Could you check a few things on this model? Use its own coordinates, in mm. Face numbers are marked on the shaded views. A direction names the side the tool comes from. Coordinates: 2 decimals unless noted, no trailing zeros. Order: outer loops, then holes, each group sorted by start corner. A loop starts at its lowest first (then second) coordinate and runs counter-clockwise, first axis right, second up. Notation, with made-up numbers: (42, 70.25) -> (70, 70.25) arc R17 ccw to (70, 98.25) -> close; hole circle Ø10 at (52.5, -36.5). An arc over 180 degrees is marked (long way). Put each result on its own line as item: value. Start each with the question number.
Q1. For the marked faces 1 and 2, which set-ups out of +Z, -Z, +X, -X, +Y, -Y let a thin tool reach every point of the face, with its end or its side?
Q2. We'd pull the mould along Y, two halves only. Please class the marked faces 3, 4 and 5: +Y half, -Y half, draft (parallel to the pull), parting line (faces both ways), or undercut.
Q3. If we section it at C-C (y = 27): Please give me the cut outline in (x, z) (3 decimals).
Q4. If we section it at B-B (x = 0): Please give me the cut outline in (y, z) (3 decimals), and give its area (3 significant figures).
Q5. Will these pins go through, and if not, where does the flat tip stop? pin 1 (1 mm diameter, centred on y = 61.5, z = 20, fed in from +X); pin 2 (4 mm diameter, centred on y = 29, z = 8, fed in from +X); pin 3 (7.5 mm diameter, centred on x = 0, y = 90.49, fed in from +Z); pin 4 (9 mm diameter, centred on x = 0, z = 0, fed in from -Y).
Q6. If we section it at A-A (z = 0): Please give me the cut outline in (x, y) (3 decimals), and give its area (3 significant figures).
Q7. Please list where these lines run through material, in increasing order: line 1 along Y through (x, z) = (0, -9) (3 decimals); line 2 along Z through (x, y) = (0, 77); line 3 along Z through (x, y) = (-6, 31).
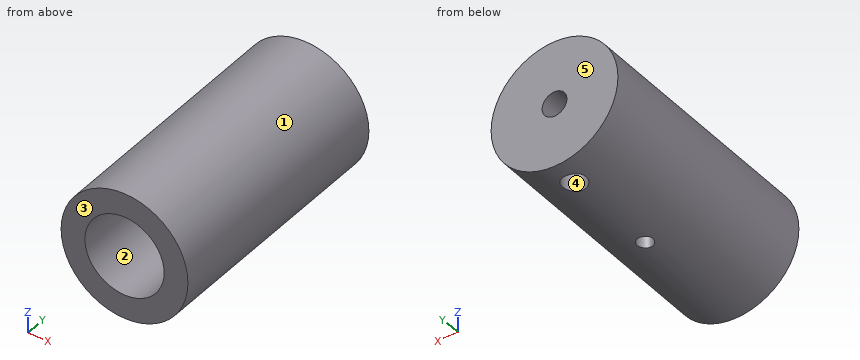
from build123d import *

# Parameters (mm, degrees)
F0_R     = 25.4
F1_DEPTH = 101.6
F2_R     = 15.875
F3_DEPTH = 50.8
F4_R     = 4.960938
F5_DEPTH = 101.601
F6_R     = 3.175
F7_DEPTH = 25.4
F8_R     = 4.7625
F9_DEPTH = 127


with BuildPart() as f1:
    # F0 (on Front) → F1 (new body)
    with BuildSketch(Plane.XZ):
        Circle(F0_R)
    extrude(amount=-F1_DEPTH)

    # F2 (on Front) → F3 (cut)
    with BuildSketch(Plane.XZ):
        Circle(F2_R)
    extrude(amount=-F3_DEPTH, mode=Mode.SUBTRACT)

    # F4 (on Front) → F5 (cut, through all)
    with BuildSketch(Plane.XZ):
        Circle(F4_R)
    extrude(amount=-F5_DEPTH, mode=Mode.SUBTRACT)

    # F6 (on Top) → F7 (cut)
    with BuildSketch(Plane.XY):
        with Locations((0, 50.8)):
            Circle(F6_R)
    extrude(amount=-F7_DEPTH, mode=Mode.SUBTRACT)

    # F8 (on Top) → F9 (cut)
    with BuildSketch(Plane.XY):
        with Locations((0, 90.4875)):
            Circle(F8_R)
    extrude(amount=-F9_DEPTH, mode=Mode.SUBTRACT)


solid = f1.part
The answers:
1. face 1: +Y, -Y
1. face 2: -Y
2. face 3: -Y half
2. face 4: undercut
2. face 5: +Y half
3. outline: circle Ø50.8 at (0, 0); hole circle Ø31.75 at (0, 0)
4. outline: (0, -25.4) -> (47.625, -25.4) -> (47.625, -15.875) -> (0, -15.875) -> close; (0, 15.875) -> (50.8, 15.875) -> (50.8, 4.961) -> (101.6, 4.961) -> (101.6, 25.4) -> (0, 25.4) -> close; (53.975, -25.4) -> (85.725, -25.4) -> (85.725, -4.961) -> (53.975, -4.961) -> close; (95.25, -25.4) -> (101.6, -25.4) -> (101.6, -4.961) -> (95.25, -4.961) -> close
4. area: 2,750 mm^2
5. pin 1: x = 16.28
5. pin 2: x = 24.68
5. pin 3: z = 25.4
5. pin 4: through
6. outline: (-25.4, 0) -> (-15.875, 0) -> (-15.875, 50.8) -> (-4.961, 50.8) -> (-4.961, 101.6) -> (-25.4, 101.6) -> close; (4.961, 50.8) -> (15.875, 50.8) -> (15.875, 0) -> (25.4, 0) -> (25.4, 101.6) -> (4.961, 101.6) -> close
6. area: 3,040 mm^2
7. line 1: 53.975 to 85.725, 95.25 to 101.6
7. line 2: -25.4 to -4.96, 4.96 to 25.4
7. line 3: -24.68 to -14.7, 14.7 to 24.68
